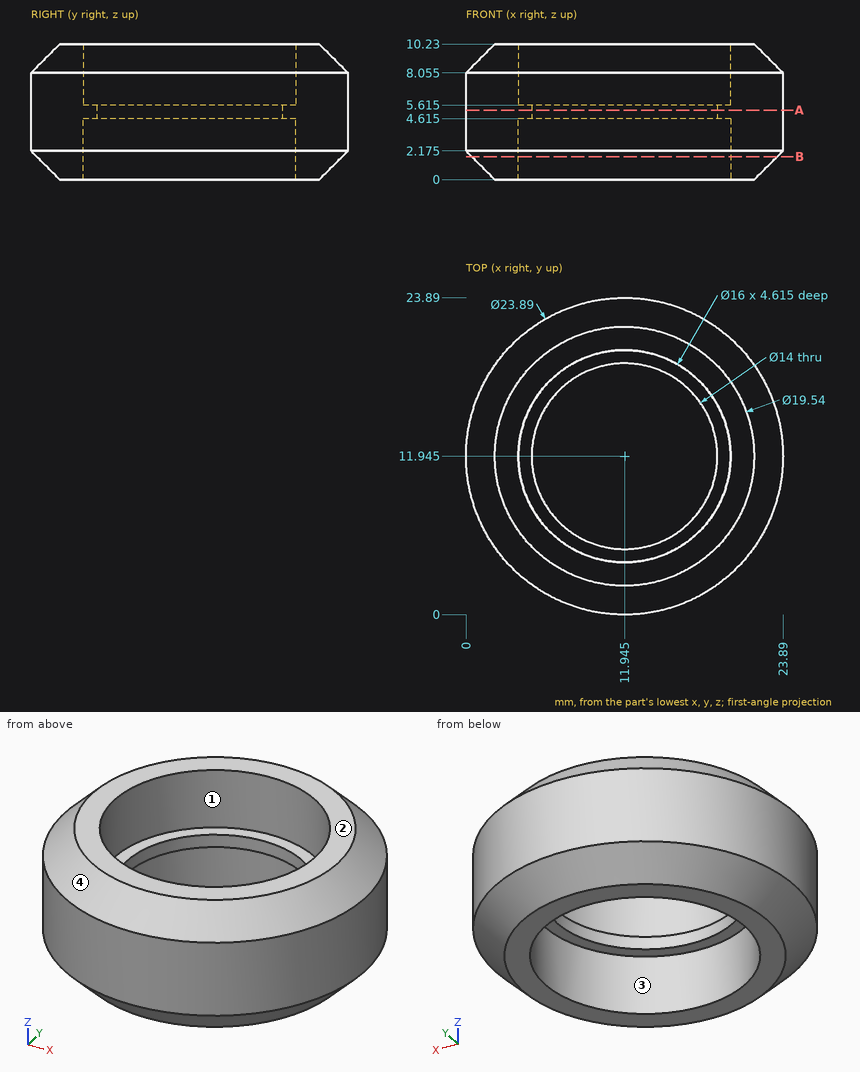
For this review, use the dimensioned drawing (mm, ordinates from the lowest corner) and the shaded views. Round coordinates to 2 decimals unless told otherwise and drop trailing zeros. Write each loop counter-clockwise with the first axis right and the second up, starting at its lowest first coordinate (ties: lowest second). Pieces come first, ordered by that corner, then holes. Notation, with made-up numbers: M 33,-15.75 L 41,-15.75 A11 ccw 41,-0.75 Z; hole C -22,12.5 d5. An arc over 180 degrees is marked long. Write item = value, one per line. Start each with the question number.
(1) Clearance check with flat-ended pins moving along their axes: pin 1 Ø2 at (y, z) = (20, 9) entering from +X; pin 2 Ø2 at (y, z) = (5.5, 7) entering from +X. State where each tip first meets the part, or that it passes through.
(2) The part is to be moulded in two halves that separate along Y. For the marked faces 1, 2, 3 and 4, say which applies: +Y half, -Y half, draft (parallel to the pull), parting line (faces both ways), or undercut.
(3) We need section B-B (z = 1.75). Give the boundary of the cut face in (x, y) (3 decimals).
(4) For line 1 along Y through (x, z) = (11.75, 6.25); line 2 along X through (y, z) = (18.25, 1.5), list the stretches that pass through material, from the lowest coordinate up.
(5) We need section A-A (z = 5.25). Give the boundary of the cut face in (x, y) (3 decimals), then the cut area to 3 significant figures.
Results found:
q1.pin_1 = 21.1
q1.pin_2 = 22.58
q2.face_1 = undercut
q2.face_2 = draft
q2.face_3 = undercut
q2.face_4 = parting line
q3.outline = C 11.945,11.945 d23.04; hole C 11.945,11.945 d16
q4.line_1 = 0 to 3.95, 19.94 to 23.89
q4.line_2 = 2.6 to 7.02, 16.87 to 21.29
q5.outline = C 11.945,11.945 d23.89; hole C 11.945,11.945 d14
q5.area = 294 mm²
